The model under review builds one solid part; all positions refer to its coordinate system, in mm. A direction names the side the tool comes from. Give positions to 0.01 mm unless a question says otherwise; leave off trailing zeros. Order: outer loops, then holes, each group sorted by start corner. A loop starts at its lowest first (then second) coordinate and runs counter-clockwise, first axis right, second up. Notation, with made-up numbers: (67, 2.5) - (96, 2.5) arc R20 cw to (96, 22.5) - close; hole circle Ø4 at (48, -6). An arc over 180 degrees is marked (long way). Use CSV: the item, a comma, the result in double quotes. Start each with the question number.
```python
from build123d import *

# Parameters (mm, degrees)
F0_W     = 273.05
F0_H     = 114.3
F0_R     = 25.4
F1_DEPTH = 19.05
F3_DEPTH = 25.4
F5_DEPTH = 25.4


with BuildPart() as f1:
    # F0 (on Front) → F1 (new body)
    with BuildSketch(Plane.XZ):
        with Locations((136.525, 57.15)):
            Rectangle(F0_W, F0_H)
        with Locations((47.625, 50.8)):
            Circle(F0_R, mode=Mode.SUBTRACT)
        with Locations((225.425, 50.8)):
            Circle(F0_R, mode=Mode.SUBTRACT)
    extrude(amount=F1_DEPTH)

    # F2 (on face) → F3 (cut)
    with BuildSketch(Plane.XZ.offset(19.05)):
        with BuildLine():
            Line((177.8, 114.3), (95.25, 114.3))
            Line((95.25, 114.3), (95.25, 55.88))
            ThreePointArc((95.25, 55.88), (98.597769, 47.797769), (106.68, 44.45))
            Line((106.68, 44.45), (166.37, 44.45))
            ThreePointArc((166.37, 44.45), (174.452231, 47.797769), (177.8, 55.88))
            Line((177.8, 55.88), (177.8, 114.3))
        make_face()
    extrude(amount=-F3_DEPTH, mode=Mode.SUBTRACT)

    # F4 (on face) → F5 (cut)
    with BuildSketch(Plane.XZ.offset(19.05)):
        Polygon((166.37, 33.364765), (166.37, 44.45), (148.622125, 44.45), (148.622125, 33.364765), (66.095858, 33.364765), (47.032329, 25.406915), (219.736259, 26.045238), (206.231396, 34.163728), align=None)
    extrude(amount=-F5_DEPTH, mode=Mode.SUBTRACT)


solid = f1.part
```
1. Clearance check with a flat-ended pin moving along its axis: pin 1 (9.5 mm diameter, centred on x = 130.5, y = -8, fed in from +Z). State where the tip first meets the part, or that it passes through.
2. Consider section A-A (z = 79). Give the boundary of the cut face in (x, y), and give its area (3 significant figures).
3. Consider section C-C (z = 50.8). Give the boundary of the cut face in (x, y) (3 decimals).
4. To check wall thickness, follow L1, parallel to X at y = -5.5, z = 50.8 (3 decimals); L2, parallel to X at y = -2.5, z = 71; L3, parallel to X at y = -9.5, z = 84. State the ranges of each line that lie inside material, in increasing order. Write a range as [from, to].
5. Consider section B-B (x = 70). Give the boundary of the cut face in (y, z), and give its area (3 significant figures).
6. Tool access review of faces 4 (the face through (108, -10, 33.365)), 5 (the face through (135, -9, 0)), 6 (the face through (98.509, -9.658, 47.887)): name each direction out of +Z, -Z, +X, -X, +Y, -Y from which nothing blocks a thin tool from reaching the whole face with its end or side.
7. Mouldability with a two-part tool opening along Z and no side actions: class faces 1 (the face through (273.05, -9, 56)), 2 (the face through (239.363, -9.392, 72.035)), 3 (the face through (47, -9, 114.3)) as pulls with the +Z half, pulls with the -Z half, needs draft (parallel to the pull), parting line crosses it, or undercut.
Answers follow:
1,pin 1,"stops at z = 44.45"
2,outline,"(0, -19.05) - (95.25, -19.05) - (95.25, 0) - (0, 0) - close; (177.8, -19.05) - (273.05, -19.05) - (273.05, 0) - (177.8, 0) - close"
2,area,"3,630 mm^2"
3,outline,"(0, -19.05) - (22.225, -19.05) - (22.225, 0) - (0, 0) - close; (73.025, -19.05) - (96.441, -19.05) - (96.441, 0) - (73.025, 0) - close; (176.609, -19.05) - (200.025, -19.05) - (200.025, 0) - (176.609, 0) - close; (250.825, -19.05) - (273.05, -19.05) - (273.05, 0) - (250.825, 0) - close"
4,L1,"x = [0, 22.225], [73.025, 96.441], [176.609, 200.025], [250.825, 273.05]"
4,L2,"x = [0, 32.23], [63.02, 95.25], [177.8, 210.03], [240.82, 273.05]"
4,L3,"x = [0, 95.25], [177.8, 273.05]"
5,outline,"(-19.05, 0) - (0, 0) - (0, 25.49) - (-19.05, 25.49) - close; (-19.05, 33.36) - (0, 33.36) - (0, 38.78) - (-19.05, 38.78) - close; (-19.05, 62.82) - (0, 62.82) - (0, 114.3) - (-19.05, 114.3) - close"
5,area,"1,570 mm^2"
6,face 4,"+Y, -Y"
6,face 5,"-Z, +X, -X, +Y, -Y"
6,face 6,"+Z, +Y, -Y"
7,face 1,"needs draft"
7,face 2,"undercut"
7,face 3,"pulls with the +Z half"
